Autodesk Inventor part; units mm, degrees
ref_plane "作業平面1" through (8.75, 0, 15.5) normal (1, 0, 0) x (0, 0, -1)
ref_plane "作業平面2" through (-8.75, 0, 11.5) normal (1, 0, 0) x (0, 0, -1)
ref_plane "YZ Plane" through (0, 0, 0) normal (1, 0, 0) x (0, 1, 0)
sketch "スケッチ1" plane through (0, 0, 0) normal (0, 1, 0) x (-1, 0, 0)
  line L0 (6.25, 11.5) -> (-6.25, 11.5)
  line L1 (-6.25, 11.5) -> (-6.25, -11.5)
  line L2 (-6.25, -11.5) -> (6.25, -11.5)
  line L3 (6.25, -11.5) -> (6.25, 11.5)
  line L4 (6.25, -11.5) -> (-6.25, 11.5) construction
  line L5 (6.25, 11.5) -> (-6.25, -11.5) construction
  line L6 (11.25, 11.5) -> (11.25, -11.5)
  line L7 (-11.25, 11.5) -> (-11.25, -11.5)
  line L8 (0, 4) -> (0, -4) construction
  line L9 (0, 14) -> (0, -14) construction
  line L10 (11.25, -11.5) -> (11.25, -15.5)
  line L11 (11.25, -15.5) -> (-11.25, -15.5)
  line L12 (-11.25, -15.5) -> (-11.25, -11.5)
  line L13 (-11.25, 11.5) -> (-11.25, 15.5)
  line L14 (-11.25, 15.5) -> (11.25, 15.5)
  line L15 (11.25, 15.5) -> (11.25, 11.5)
  point P0 (0, 0)
  point P1 (0, 0)
  point P2 (0, 0)
  point P3 (0, -14)
  dimension "d0" = 23
  dimension "d1" = 12.5
  dimension "d2" = 5
  dimension "d3" = 28
  dimension "d4" = 8
  dimension "d21" = 4
  dimension "d26" = 5
  dimension "d27" = 4
extrude "押し出し1" add sketch "スケッチ1" along normal blind 2
hole "穴1" at (0, 0, 4) at (0, 0, -4) at (0, 0, 14) at (0, 0, -14) direction (0, 1, 0) diameter 1.5 end through all
sketch "スケッチ2" plane through (0, 2, 0) normal (0, 1, 0) x (1, 0, 0)
  line L0 (-6.25, -11.5) -> (-6.25, 11.5)
  circle A0 centre (0, -14) radius 0.75
  circle A1 centre (0, 14) radius 0.75
  line L1 (-11.25, 15.5) -> (-11.25, -15.5)
  line L2 (11.25, -15.5) -> (11.25, 15.5)
  line L3 (11.25, 15.5) -> (-11.25, 15.5)
  line L4 (-11.25, -15.5) -> (11.25, -15.5)
  line L5 (-11.25, 15.5) -> (-11.25, -15.5)
  line L6 (-11.25, -15.5) -> (11.25, -15.5)
  line L7 (-6.25, -15.5) -> (-11.25, -15.5)
  line L8 (-11.25, -15.5) -> (-11.25, -10.5)
  line L9 (-11.25, -10.5) -> (-6.25, -10.5)
  line L10 (-6.25, -10.5) -> (-6.25, -15.5)
  line L11 (6.25, -11.5) -> (-6.25, -11.5)
  line L12 (-6.25, -11.5) -> (-6.25, 11.5)
  line L13 (-6.25, 11.5) -> (6.25, 11.5)
  line L14 (6.25, 11.5) -> (6.25, -11.5)
  point P0 (0, 0)
  point P1 (-6.25, -10.5)
  dimension "d28" = 5
extrude "押し出し2" add sketch "スケッチ2" along normal blind 5 contours L10 L4 L1 L9 L0
sketch "スケッチ6" plane through (-6.25, 2, 10.5) normal (0, 0, -1) x (-1, 0, 0)
  line L0 (5, 0) -> (0, 5) construction
  line L1 (5, 5) -> (0, 0) construction
  circle A0 centre (2.5, 2.5) radius 1.25
  point P0 (-6.25, -2)
  dimension "d29" = 2.5
extrude "押し出し5" cut sketch "スケッチ6" along normal through all both and the other way through all
mirror "ミラー4" about plane through (0, 0, 0) normal (0, 0, 1) of "押し出し2", "押し出し5"
sketch "スケッチ7" plane through (0, 2, 0) normal (0, 1, 0) x (1, 0, 0)
  line L0 (-6.25, 10.5) -> (-11.25, 10.5)
  line L1 (-11.25, -10.5) -> (-6.25, -10.5)
  line L2 (-6.25, -10.5) -> (-11.25, 10.5) construction
  line L3 (-6.25, 10.5) -> (-11.25, -10.5) construction
  line L4 (-7.75, -10.5) -> (-9.75, -10.5)
  line L5 (-9.75, -10.5) -> (-9.75, 10.5)
  line L6 (-9.75, 10.5) -> (-7.75, 10.5)
  line L7 (-7.75, 10.5) -> (-7.75, -10.5)
  line L8 (-7.75, -10.5) -> (-9.75, 10.5) construction
  point P0 (0, 0)
  point P1 (-8.75, 0)
  dimension "d32" = 2
extrude "押し出し6" cut sketch "スケッチ7" against normal through all
mirror "ミラー5" about plane through (0, 0, 0) normal (1, 0, 0) of "押し出し2", "押し出し5", "ミラー4", "押し出し6"
fillet "フィレット1" radius 1.2 8 edges at (-10.5, 2, -10.5) (-7, 2, -10.5) (7, 2, -10.5) (10.5, 2, -10.5) (-10.5, 2, 10.5) (-7, 2, 10.5) (7, 2, 10.5) (10.5, 2, 10.5)
ref_plane "作業平面1" through (8.75, 0, 15.5) normal (1, 0, 0) x (0, 0, -1)
ref_plane "作業平面2" through (-8.75, 0, 11.5) normal (1, 0, 0) x (0, 0, -1)
equation "\"d26\" = d2"
equation "\"d27\" = d21"
properties part number "om_DropBase_8g" material "ABS プラスチック"
Verification items for the finished model (mm, model axes). A direction names the side the tool comes from. Coordinates: 2 decimals unless noted, no trailing zeros. Order: outer loops, then holes, each group sorted by start corner. A loop starts at its lowest first (then second) coordinate and runs counter-clockwise, first axis right, second up. Notation, with made-up numbers: (49, -38) -> (62, -38) arc R24 cw to (62, -7) -> close; hole circle Ø6 at (47, -15.5). An arc over 180 degrees is marked (long way). Put each result on its own line as item: value. Start each with the question number.
1. Cross-section at D-D, the plane y = 6.5. Record the boundary of the cut face in (x, z).
2. Cross-section at B-B, the plane x = -4.25. Record the boundary of the cut face in (y, z).
3. Go/stop test with a flat-tipped pin: pin 1 Ø0.8 at (x, z) = (-7, -2.5) entering from +Y. Record where the tip stops, or that it passes through.
4. Mould release check, pull along Z, two halves, no side actions. Record for faces 5 (the flat face through (-7, 0, 0)), 6 (the flat face through (0, 1, 15.5)), 7 (the flat face through (8, 3, 10.5)): released by +Z, released by -Z, zero draft, split by the parting line, or undercut.
5. Cross-section at C-C, the plane z = 3. Record the boundary of the cut face in (x, y).
6. Access from +Z, -Z, +X, -X, +Y, -Y to the whole of each face (thin tool, end or side, straight path). Record for faces 1 (the flat face through (-8, 3, -10.5)), 2 (the flat face through (-10, 2, 0)), 3 (the flat face through (0, 1, 11.5)), 4 (the flat face through (-9, 7, -13)).
7. Material ranges on L1, parallel to Z at x = 0, y = 1.5; L2, parallel to X at y = 1.25, z = 2; L3, parallel to X at y = 0.85, z = -14, recorded low to high. Write a range as [from, to].
8. Cross-section at A-A, the plane z = 14. Record the boundary of the cut face in (x, y), then the cut area to 3 significant figures.
Computed:
1. outline: (-11.25, -15.5) -> (-6.25, -15.5) -> (-6.25, -10.5) -> (-11.25, -10.5) -> close; (-11.25, 10.5) -> (-6.25, 10.5) -> (-6.25, 15.5) -> (-11.25, 15.5) -> close; (6.25, -15.5) -> (11.25, -15.5) -> (11.25, -10.5) -> (6.25, -10.5) -> close; (6.25, 10.5) -> (11.25, 10.5) -> (11.25, 15.5) -> (6.25, 15.5) -> close
2. outline: (0, -15.5) -> (2, -15.5) -> (2, -11.5) -> (0, -11.5) -> close; (0, 11.5) -> (2, 11.5) -> (2, 15.5) -> (0, 15.5) -> close
3. pin 1: y = 2
4. face 5: zero draft
4. face 6: released by +Z
4. face 7: undercut
5. outline: (-11.25, 0) -> (-9.75, 0) -> (-9.75, 2) -> (-11.25, 2) -> close; (-7.75, 0) -> (-6.25, 0) -> (-6.25, 2) -> (-7.75, 2) -> close; (6.25, 0) -> (7.75, 0) -> (7.75, 2) -> (6.25, 2) -> close; (9.75, 0) -> (11.25, 0) -> (11.25, 2) -> (9.75, 2) -> close
6. face 1: +Y
6. face 2: +X, -X, +Y
6. face 3: +Y, -Y
6. face 4: +Z, -Z, +X, -X, +Y
7. L1: [-15.5, -14.75], [-13.25, -11.5], [11.5, 13.25], [14.75, 15.5]
7. L2: [-11.25, -9.75], [-7.75, -6.25], [6.25, 7.75], [9.75, 11.25]
7. L3: [-11.25, -0.75], [0.75, 11.25]
8. outline: (-11.25, 0) -> (-0.75, 0) -> (-0.75, 2) -> (-6.25, 2) -> (-6.25, 7) -> (-11.25, 7) -> close; (0.75, 0) -> (11.25, 0) -> (11.25, 7) -> (6.25, 7) -> (6.25, 2) -> (0.75, 2) -> close; hole circle Ø2.5 at (-8.75, 4.5); hole circle Ø2.5 at (8.75, 4.5)
8. area: 82.2 mm2
